Check sheet for the modelled part. Datum: model origin and axes. Units: mm. A direction names the side the tool comes from. Give positions to 0.01 mm unless a question says otherwise; leave off trailing zeros. Write each loop counter-clockwise with the first axis right and the second up, starting at its lowest first coordinate (ties: lowest second). Pieces come first, ordered by that corner, then holes. Notation, with made-up numbers: M -34.5,56.5 L -20.5,56.5 A18 cw -20.5,89.5 Z; hole C 81,15 d6. An arc over 180 degrees is marked long. Write each question's results on one line, items separated by ' | '. Start each with the question number.
from build123d import *

# Parameters (mm, degrees)
SKETCH8_R           = 6.3246
BOSS_EXTRUDE7_DEPTH = 127
SKETCH9_W           = 3.175
SKETCH9_H           = 1.6002
BOSS_EXTRUDE8_DEPTH = 49.911
SKETCH10_W          = 21.336
SKETCH10_H          = 1.002575458
CUT_EXTRUDE1_DEPTH  = 3.937
CUT_EXTRUDE2_DEPTH  = 8.89


with BuildPart() as part:
    # Sketch8 → Boss-Extrude7 (new body)
    with BuildSketch(Plane.XY):
        Circle(SKETCH8_R)
    extrude(amount=BOSS_EXTRUDE7_DEPTH)

    # Sketch9 → Boss-Extrude8 (add)
    with BuildSketch(Plane.XY):
        with Locations((0, -6.3246)):
            Rectangle(SKETCH9_W, SKETCH9_H)
    extrude(amount=BOSS_EXTRUDE8_DEPTH)

    # Sketch10 → Cut-Extrude1 (cut)
    with BuildSketch(Plane.ZY.offset(1.5875)):
        with Locations((10.668, -6.623412271)):
            Rectangle(SKETCH10_W, SKETCH10_H)
    extrude(amount=-CUT_EXTRUDE1_DEPTH, mode=Mode.SUBTRACT)

    # Sketch11 → Cut-Extrude2 (cut)
    with BuildSketch(Plane.XY.offset(127)):
        Polygon((4.7625, 0), (2.38125, 4.124445986), (-2.38125, 4.124445986), (-4.7625, 0), (-2.38125, -4.124445986), (2.38125, -4.124445986), align=None)
    extrude(amount=-CUT_EXTRUDE2_DEPTH, mode=Mode.SUBTRACT)


solid = part.part
Q1. Section check B-B on y = 2.5. Record the boundary of the cut face in (x, z).
Q2. Release check for a two-part mould opening along Y. For faces 1 (the face through (0, -7.125, 35)), 2 (the face through (3.4, 5.333, 62.611)), 3 (the face through (0, 4.124, 123)), 4 (the face through (0, 0, 0)) record: pulls with the +Y half, pulls with the -Y half, needs draft (parallel to the pull), parting line crosses it, or undercut.
Q3. Tool access check on faces 5 (the face through (3.59, 2.03, 122.62)), 6 (the face through (4.1, 1.5, 127)), 7 (the face through (0, -6.122, 11)). Record the directions out of +Z, -Z, +X, -X, +Y, -Y that give a thin tool (end or side, any length) a straight path to the whole face; none if there is none.
Q4. Depth check by flat-ended pin: pin 1 Ø2 at (x, z) = (-4.5, 42.5) entering from -Y; pin 2 Ø6.5 at (x, y) = (-1, 1) entering from +Z; pin 3 Ø2.5 at (x, z) = (0, 8.5) entering from -Y; pin 4 Ø3 at (y, z) = (-3.5, 110.5) entering from +X. Enter the tip coordinate at first touch or a pass-through.
Q5. Section check A-A on x = 0. Record the boundary of the cut face in (y, z).
Q6. Section check C-C on z = 70. Record the boundary of the cut face in (x, y), plus the area to 3 significant figures.
Q7. Scan lines: L1, parallel to X at y = -0.5, z = 67; L2, parallel to Z at x = -0.5, y = 3.75; L3, parallel to Y at x = -0.5, z = 17. Record each from-to range of solid material in increasing order.
Check result:
1) outline: M -5.81,0 L 5.81,0 L 5.81,127 L 3.32,127 L 3.32,118.11 L -3.32,118.11 L -3.32,127 L -5.81,127 Z
2) face 1: pulls with the -Y half | face 2: parting line crosses it | face 3: undercut | face 4: needs draft
3) face 5: +Z | face 6: +Z, +X, -X, +Y, -Y | face 7: -Z, +X, -X, -Y
4) pin 1: y = -5.27 | pin 2: z = 127 | pin 3: y = -6.12 | pin 4: x = 6
5) outline: M -7.12,21.34 L -6.12,21.34 L -6.12,0 L 6.32,0 L 6.32,127 L 4.12,127 L 4.12,118.11 L -4.12,118.11 L -4.12,127 L -6.32,127 L -6.32,49.91 L -7.12,49.91 Z
6) outline: C 0,0 d12.65 | area: 126 mm^2
7) L1: -6.3 to 6.3 | L2: 0 to 118.11 | L3: -6.12 to 6.3
